from build123d import *

# Parameters (mm, degrees)
SZKIC2_R                   = 6
WYTNIJ_WYCI_GNI_CIE1_DEPTH = 28


with BuildPart() as part:
    # Szkic1 → Obrót1 (revolve)
    with BuildSketch(Plane(origin=(0, 0, 0), x_dir=(1, 0, 0), z_dir=(0, 1, 0)), mode=Mode.PRIVATE) as obr_t1_sk:
        Polygon((-14, 6), (-17.5, 6), (-17.5, 9), (-14, 9), (-14, 16.1), (14, 16.1), (14, 9), (17.5, 9), (17.5, 6), (14, 6), (14, 0), (-14, 0), align=None)
    revolve(obr_t1_sk.sketch.rotate(Axis((-14, 0, 0), (1, 0, 0)), 180), axis=Axis((-14, 0, 0), (1, 0, 0)))

    # Szkic2 → Wytnij-wyciągnięcie1 (cut)
    with BuildSketch(Plane.ZY.offset(14)):
        Circle(SZKIC2_R)
    extrude(amount=-WYTNIJ_WYCI_GNI_CIE1_DEPTH, mode=Mode.SUBTRACT)


solid = part.part
The listing builds one solid part. Answer for the finished solid, in the listing's coordinates (mm). A direction names the side the tool comes from. Coordinates: 2 decimals unless noted, no trailing zeros. Order: outer loops, then holes, each group sorted by start corner. A loop starts at its lowest first (then second) coordinate and runs counter-clockwise, first axis right, second up. Notation, with made-up numbers: (5, 46.25) -> (44, 46.25) arc R13 cw to (44, 60.25) -> close; hole circle Ø2 at (-37, 15). An arc over 180 degrees is marked (long way). Answer in a Markdown table with one row per item. Add a question column.
Item 1: Determine the mould class of faces 4 (the face through (17.5, 6, 2)), 5 (the face through (-15.726, -6.083, -6.633)), 6 (the face through (-0.245, -1.802, 5.723)) for opening direction Z: +Z half, -Z half, draft (parallel to the pull), parting line (faces both ways), or undercut.
Item 2: Find section D-D (y = -6.5). Write down the section's boundary in (x, z).
Item 3: Find the intervals of material crossed by L1, parallel to Y at x = 6, z = 0; L2, parallel to X at y = 6.5, z = -8; L3, parallel to Y at x = 11, z = -2, in increasing order. Write a range as from..to.
Item 4: Which of the six approach directions +Z, -Z, +X, -X, +Y, -Y give full straight-line access (tool end or side, diameter ignored) to faces 1 (the face through (14, 7, 7)), 2 (the face through (-17.5, 6, -2)), 3 (the face through (-14, 7, -7))?
Item 5: Find section A-A (y = 0). Write down the section's boundary in (x, z).
Item 6: Each of these flat-tipped pins is pushed along its axis until it touches: P1, Ø5, axis at x = 9, y = -7.5, coming from the +Z side; P2, Ø10, axis at x = -1, z = -6, coming from the +Y side; P3, Ø1, axis at x = -2.5, y = 1.5, coming from the -Z side. Where does it stop, or does it pass through?
Item 7: Find section C-C (x = -9.5). Write down the section's boundary in (y, z).
Result set:
| question | item | result |
|---|---|---|
| 1 | face 4 | draft |
| 1 | face 5 | parting line |
| 1 | face 6 | undercut |
| 2 | outline | (-17.5, -6.22) -> (-14, -6.22) -> (-14, -14.73) -> (14, -14.73) -> (14, -6.22) -> (17.5, -6.22) -> (17.5, 6.22) -> (14, 6.22) -> (14, 14.73) -> (-14, 14.73) -> (-14, 6.22) -> (-17.5, 6.22) -> close |
| 3 | L1 | y = -16.1..-6, 6..16.1 |
| 3 | L2 | x = -14..14 |
| 3 | L3 | y = -15.98..-5.66, 5.66..15.98 |
| 4 | face 1 | +X |
| 4 | face 2 | +Z, -Z, -X, +Y, -Y |
| 4 | face 3 | -X |
| 5 | outline | (-17.5, -9) -> (-14, -9) -> (-14, -16.1) -> (14, -16.1) -> (14, -9) -> (17.5, -9) -> (17.5, -6) -> (-17.5, -6) -> close; (-17.5, 6) -> (17.5, 6) -> (17.5, 9) -> (14, 9) -> (14, 16.1) -> (-14, 16.1) -> (-14, 9) -> (-17.5, 9) -> close |
| 6 | P1 | stops at z = 15.3 |
| 6 | P2 | stops at y = 16.07 |
| 6 | P3 | stops at z = -16.07 |
| 7 | outline | circle Ø32.2 at (0, 0); hole circle Ø12 at (0, 0) |
